Input: part model. Units: mm. Frame: model coordinates. A direction names the side the tool comes from. Round coordinates to 2 decimals unless told otherwise and drop trailing zeros. Order: outer loops, then holes, each group sorted by start corner. A loop starts at its lowest first (then second) coordinate and runs counter-clockwise, first axis right, second up. Notation, with made-up numbers: (-39.5, 35) -> (-3.5, 35) arc R18 ccw to (-3.5, 43) -> close; hole circle Ø5 at (42.25, 18). An arc over 180 degrees is marked (long way). Use a Markdown table: item, result.
Solid Edge part; units mm, degrees
sketch "Sketch1" plane through (0, 0, 0) normal (0, -1, 0) x (1, 0, 0)
  line L0 (4, 0) -> (1.8, 0)
  line L1 (1.8, 0) -> (1.8, -1.4)
  line L2 (1.8, -1.4) -> (2, -1.4)
  line L3 (2, -1.4) -> (2, -40)
  line L4 (2, -40) -> (0, -40)
  arc A0 (0, 3.1) -> (4, 2.0282) centre (0, -4.9) cw
  line L5 (4, 0) -> (4, 2.0282)
  dimension "D1" = 1.8
  dimension "D2" = 1.8
revolve "RevolvedProtrusion1" add sketch "Sketch1" angle 360 about axis through (0, 0, -6) along (0, 0, 1)
cosmetic_thread "Thread1"
chamfer "Chamfer_1" distance 0.4 angle 45 1 edges at (-2, 0, -40)
fillet "Round1" radius 0.2 2 edges at (-1.8, 0, -1.4) (-1.8, 0, 0)
fillet "Round_3" radius 1 1 edges at (-4, 0, 2.0282)
sketch "Sketch2" plane through (0, 0, 3.1) normal (0, 0, 1) x (1, 0, 0)
  line L0 (-0.5, 0.5) -> (-0.5, 2.3)
  line L1 (-0.5, 2.3) -> (0.5, 2.3)
  line L2 (0.5, 2.3) -> (0.5, 0.5)
  line L3 (0.5, 0.5) -> (2.3, 0.5)
  line L4 (2.3, 0.5) -> (2.3, -0.5)
  line L5 (2.3, -0.5) -> (0.5, -0.5)
  line L6 (0.5, -0.5) -> (0.5, -2.3)
  line L7 (0.5, -2.3) -> (-0.5, -2.3)
  line L8 (-0.5, -2.3) -> (-0.5, -0.5)
  line L9 (-0.5, -0.5) -> (-2.3, -0.5)
  line L10 (-2.3, -0.5) -> (-2.3, 0.5)
  line L11 (-2.3, 0.5) -> (-0.5, 0.5)
  dimension "D1" = 0.5
extrude "ExtrudedCutout_2" cut sketch "Sketch2" against normal blind 2.3
properties material "Galvanized steel"
1) Set-up query: faces 5 (the face through (0, 0, -40)), 6 (the face through (-0.5, 1, 2)), 7 (the face through (0, 2, -21)), 8 (the face through (1.717, -0.541, -0.707)). Return all of +Z, -Z, +X, -X, +Y, -Y with unobstructed straight access to the full face (end or side cutting, diameter ignored); none if empty.
Answer key:
| item | result |
|---|---|
| face 5 | -Z, +X, -X, +Y, -Y |
| face 6 | +Z |
| face 7 | -Z |
| face 8 | none |
2) Draft query along X for faces 1 (the face through (0, 0, 0.8)), 2 (the face through (0, 2.3, 2)), 3 (the face through (-2, -1, 0)), 4 (the face through (-0.867, -3.905, 0.722)). Return one class per face: released by +X, released by -X, zero draft, split by the parting line, or undercut.
Answer key:
| item | result |
|---|---|
| face 1 | undercut |
| face 2 | undercut |
| face 3 | zero draft |
| face 4 | split by the parting line |
3) Contact query for flat-ended pins moving along their axis: P1, Ø2, axis at x = -2, z = 2, coming from the -Y side; P2, Ø3, axis at x = -2.5, y = -2, coming from the -Z side; P3, Ø1.4, axis at y = 1.5, z = 2.5, coming from the +X side. Output: stop coordinate, or through.
Answer key:
| item | result |
|---|---|
| P1 | stops at y = -3.84 |
| P2 | stops at z = -39.9 |
| P3 | stops at x = 3.71 |
4) Cut plane A-A on z = -20.5. Return loops of the section in (x, y).
Answer key:
| item | result |
|---|---|
| outline | circle Ø4 at (0, 0) |
5) Ray query, probe 1 along Y at (x, z) = (-2, 1); probe 2 along Z at (x, y) = (0.25, -1.5); probe 3 along Y at (x, z) = (-0.25, -23.5). Return the intervals inside material, ascending.
Answer key:
| item | result |
|---|---|
| probe 1 | y = -3.46 to -0.5, 0.5 to 3.46 |
| probe 2 | z = -40 to 0.8 |
| probe 3 | y = -1.98 to 1.98 |
